```python
from build123d import *

# Parameters (mm, degrees)
SKETCH1_W              = 79.57
SKETCH1_H              = 22.8
SKETCH1_R              = 1.65
BOSS_EXTRUDE2_DEPTH    = 1.62
SKETCH2_W              = 15
SKETCH2_H              = 15
BOSS_EXTRUDE3_DEPTH    = 6.8
SKETCH3_W              = 0.65
SKETCH3_H              = 0.65
BOSS_EXTRUDE4_DEPTH    = 9.16
SKETCH4_W              = 7.72
SKETCH4_H              = 2.42
SKETCH4_W_2            = 5.07
SKETCH4_H_2            = 2.424
BOSS_EXTRUDE5_DEPTH    = 3
SKETCH5_W              = 20
SKETCH5_H              = 16
BOSS_EXTRUDE6_DEPTH    = 2.3
SKETCH6_R              = 0.45
HOLE_FOR_ANTENNA_DEPTH = 2.8
SKETCH7_R              = 0.6
BOSS_EXTRUDE7_DEPTH    = 80


with BuildPart() as part:
    # Sketch1 → Boss-Extrude2 (new body)
    with BuildSketch(Plane(origin=(0, 0, 0), x_dir=(1, 0, 0), z_dir=(0, 1, 0))):
        with Locations((39.785, 11.4)):
            Rectangle(SKETCH1_W, SKETCH1_H)
        with Locations((2.65, 11.4)):
            Circle(SKETCH1_R, mode=Mode.SUBTRACT)
        with Locations((76.92, 11.4)):
            Circle(SKETCH1_R, mode=Mode.SUBTRACT)
    extrude(amount=BOSS_EXTRUDE2_DEPTH)

    # Sketch2 → Boss-Extrude3 (add)
    with BuildSketch(Plane(origin=(0, 1.62, 0), x_dir=(1, 0, 0), z_dir=(0, 1, 0))):
        with Locations((51.68, 11.7)):
            Rectangle(SKETCH2_W, SKETCH2_H)
    extrude(amount=BOSS_EXTRUDE3_DEPTH)

    # Sketch3 → Boss-Extrude4 (add)
    with BuildSketch(Plane(origin=(0, 1.62, 0), x_dir=(1, 0, 0), z_dir=(0, 1, 0))):
        with Locations((31.665, 3.525)):
            Rectangle(SKETCH3_W, SKETCH3_H)
        with Locations((34.315, 3.525)):
            Rectangle(SKETCH3_W, SKETCH3_H)
        with Locations((36.965, 3.525)):
            Rectangle(SKETCH3_W, SKETCH3_H)
        with Locations((31.665, 8.175)):
            Rectangle(SKETCH3_W, SKETCH3_H)
        with Locations((34.315, 8.175)):
            Rectangle(SKETCH3_W, SKETCH3_H)
        with Locations((31.665, 15.825)):
            Rectangle(SKETCH3_W, SKETCH3_H)
        with Locations((34.315, 15.825)):
            Rectangle(SKETCH3_W, SKETCH3_H)
    extrude(amount=BOSS_EXTRUDE4_DEPTH)

    # Sketch4 → Boss-Extrude5 (add)
    with BuildSketch(Plane(origin=(0, 1.62, 0), x_dir=(1, 0, 0), z_dir=(0, 1, 0))):
        with Locations((34.315, 3.525)):
            Rectangle(SKETCH4_W, SKETCH4_H)
        with Locations((32.99, 8.175)):
            Rectangle(SKETCH4_W_2, SKETCH4_H)
        with Locations((32.99, 15.823)):
            Rectangle(SKETCH4_W_2, SKETCH4_H_2)
    extrude(amount=BOSS_EXTRUDE5_DEPTH)

    # Sketch5 → Boss-Extrude6 (add)
    with BuildSketch(Plane(origin=(0, 1.62, 0), x_dir=(1, 0, 0), z_dir=(0, 1, 0))):
        with Locations((17.45, 12.8)):
            Rectangle(SKETCH5_W, SKETCH5_H)
    extrude(amount=BOSS_EXTRUDE6_DEPTH)

    # Sketch6 → Hole for antenna (cut)
    with BuildSketch(Plane(origin=(0, 1.62, 0), x_dir=(1, 0, 0), z_dir=(0, 1, 0))):
        with Locations((5.5, 6)):
            Circle(SKETCH6_R)
    extrude(amount=-HOLE_FOR_ANTENNA_DEPTH, mode=Mode.SUBTRACT)

    # Sketch7 → Boss-Extrude7 (add)
    with BuildSketch(Plane(origin=(0, 1.62, 0), x_dir=(1, 0, 0), z_dir=(0, 1, 0))):
        with Locations((5.5, 6)):
            Circle(SKETCH7_R)
    extrude(amount=BOSS_EXTRUDE7_DEPTH)


solid = part.part
```
Could you check a few things on this model? Use its own coordinates, in mm. A direction names the side the tool comes from. Coordinates: 2 decimals unless noted, no trailing zeros. Order: outer loops, then holes, each group sorted by start corner. A loop starts at its lowest first (then second) coordinate and runs counter-clockwise, first axis right, second up. Notation, with made-up numbers: M 16.5,-15 L 56.5,-15 A23 ccw 56.5,14 Z; hole C -34.75,37.5 d1. An arc over 180 degrees is marked long. Use one line per item in the form item = value. Start each with the question number.
1. On a 3-axis mill with a long thin cutter (end or side, diameter ignored), from which of +Z, -Z, +X, -X, +Y, -Y can I reach the whole of each face in a straight line? I mean faces 4 (the flat face through (30.455, 3, -16)), 5 (the flat face through (33, 3, -9.385)), 6 (the flat face through (33, 3, -17.035)). Say none if no direction works.
2. Please list where these lines run through material, in increasing order: line 1 (X direction, y = 1.1, z = -11.4); line 2 (Z direction, x = 76.92, y = 0.9); line 3 (X direction, y = 0.8, z = -6).
3. Suppose I cut it at B-B on z = -11.4. Write out the boundary of the cut face in (x, y), then the cut area to 3 significant figures.
4. We'd pull the mould along X, two halves only. Please class faces 1 (the flat face through (59.18, 5, -12)), 2 (the flat face through (17, 3, -20.8)), 3 (the flat face through (39, 1.62, -12)): +X half, -X half, draft (parallel to the pull), parting line (faces both ways), or undercut.
5. Suppose I cut it at D-D on y = 28. Write out the boundary of the cut face in (x, z), then the cut area to 3 significant figures.
6. For pin 1 (0.7 mm diameter, centred on x = 31.5, y = 7.5, fed in from +Z); pin 2 (1.2 mm diameter, centred on x = 32, z = -16, fed in from +Y); pin 3 (1.5 mm diameter, centred on x = 32.5, y = 2.5, fed in from -Z) (3 decimals), each with a flat end and sliding along its axis, tell me the tip position at first contact or that it passes through.
7. Suppose I cut it at C-C on x = 21. Write out the boundary of the cut face in (y, z).
8. Suppose I cut it at A-A on x = 2.65. Write out the boundary of the cut face in (y, z), then the cut area to 3 significant figures.
Geometry says:
q1.face_4 = +Z, -Z, +Y
q1.face_5 = +Y
q1.face_6 = -Z, +Y
q2.line_1 = 0 to 1, 4.3 to 75.27, 78.57 to 79.57
q2.line_2 = -22.8 to -13.05, -9.75 to 0
q2.line_3 = 0 to 5.05, 5.95 to 79.57
q3.outline = M 0,0 L 1,0 L 1,1.62 L 0,1.62 Z; M 4.3,0 L 75.27,0 L 75.27,1.62 L 59.18,1.62 L 59.18,8.42 L 44.18,8.42 L 44.18,1.62 L 27.45,1.62 L 27.45,3.92 L 7.45,3.92 L 7.45,1.62 L 4.3,1.62 Z; M 78.57,0 L 79.57,0 L 79.57,1.62 L 78.57,1.62 Z
q3.area = 266 mm^2
q4.face_1 = +X half
q4.face_2 = draft
q4.face_3 = undercut
q5.outline = C 5.5,-6 d1.2
q5.area = 1.13 mm^2
q6.pin_1 = -3.2
q6.pin_2 = 10.78
q6.pin_3 = -17.035
q7.outline = M 0,-22.8 L 1.62,-22.8 L 1.62,-20.8 L 3.92,-20.8 L 3.92,-4.8 L 1.62,-4.8 L 1.62,0 L 0,0 Z
q8.outline = M 0,-22.8 L 1.62,-22.8 L 1.62,-13.05 L 0,-13.05 Z; M 0,-9.75 L 1.62,-9.75 L 1.62,0 L 0,0 Z
q8.area = 31.6 mm^2
